For this review, take the finished solid that the model builds, in its own axes (mm). A direction names the side the tool comes from. Give positions to 0.01 mm unless a question says otherwise; leave off trailing zeros. Order: outer loops, then holes, each group sorted by start corner. A loop starts at its lowest first (then second) coordinate and runs counter-clockwise, first axis right, second up. Notation, with made-up numbers: (61, 50) - (76, 50) arc R22 ccw to (76, 72) - close; hole circle Ø3 at (-5, 29). An arc over 180 degrees is marked (long way). One line per item, written item: value.
```python
from build123d import *

# Parameters (mm, degrees)
F1_DEPTH = 100
F2_DEPTH = 25.4


with BuildPart() as f1:
    # F0 (on Top) → F1 (new body)
    with BuildSketch(Plane.XY):
        with BuildLine():
            Line((-63.4819120169, 0), (-63.4819120169, -53.9388507605))
            Line((-63.4819120169, -53.9388507605), (-13.6922001839, -17.2189325094))
            Line((-13.6922001839, -17.2189325094), (-13.6922001839, 41.2839800119))
            Line((-13.6922001839, 41.2839800119), (-37.5497788191, 41.2839800119))
            Line((-37.5497788191, 41.2839800119), (-37.5497788191, 25.9321331978))
            ThreePointArc((-37.5497788191, 25.9321331978), (-55.8865660539, 18.3367872348), (-63.4819120169, 0))
        make_face()
    extrude(amount=F1_DEPTH)

    # F2 (add): a face of the model
    f2_faces = [f1.faces().sort_by_distance(p)[0] for p in [
        (-38.5870561004, -35.5788916349, 50),
    ]]
    extrude(f2_faces, amount=F2_DEPTH)


solid = f1.part
```
(1) Take a section at A-A (z = 22). Write out the cut boundary in (x, y), then the cut area to 3 significant figures.
Answers below:
outline: (-63.48, -53.94) - (-48.41, -74.38) - (1.38, -37.66) - (-13.69, -17.22) - (-13.69, 41.28) - (-37.55, 41.28) - (-37.55, 25.93) arc R25.93 ccw to (-63.48, 0) - close
area: 4,860 mm^2
(2) Machinability: for faces 1 (the face through (-37.55, 34, 49)), 2 (the face through (-13.692, 12, 49)), 3 (the face through (-36, -11, 100)), which of the approach directions +Z, -Z, +X, -X, +Y, -Y give a long, thin tool a straight path to every point of the face, cutting with its end or side? Answer none if there is none.
Answers below:
face 1: +Z, -Z, -X, +Y
face 2: +Z, -Z, +X, +Y
face 3: +Z, +X, -X, +Y, -Y
(3) Take a section at C-C (y = -45). Write out the cut boundary in (x, z), then the cut area to 3 significant figures.
Answers below:
outline: (-63.48, 0) - (-8.57, 0) - (-8.57, 100) - (-63.48, 100) - close
area: 5,490 mm^2
(4) Wall thickness on line 1 (X direction, y = -7, z = 59); line 2 (Y direction, x = -25, z = 56); line 3 (X direction, y = -28.5, z = 71): over which ranges is each line inside the solid? List them lowest first. Write a range as from..to.
Answers below:
line 1: x = -63.48..-13.69
line 2: y = -57.12..41.28
line 3: x = -63.48..-5.37
(5) Take a section at B-B (x = -52). Write out the cut boundary in (y, z), then the cut area to 3 significant figures.
Answers below:
outline: (-69.51, 0) - (21.53, 0) - (21.53, 100) - (-69.51, 100) - close
area: 9,100 mm^2
(6) For P1, Ø6, axis at x = -34.5, z = 27, coming from the -Y side; P2, Ø10, axis at x = -8, z = 62, coming from the -Y side; P3, Ø8, axis at x = -34.5, z = 40, coming from the -Y side, all flat-tipped, find the tip position at first contact; note any pin that passes through.
Answers below:
P1: stops at y = -66.34
P2: stops at y = -48.27
P3: stops at y = -67.08
